Here's how the part is built. I have some questions about the finished solid (model axes, mm). A direction names the side the tool comes from. Coordinates: 2 decimals unless noted, no trailing zeros. Loops run counter-clockwise (first coordinate to the right, second up) from the corner with the lowest first, then second, coordinate; pieces in that order, holes last. Notation, with made-up numbers: (0.5, 73.5) -> (51.5, 73.5) arc R28 ccw to (51.5, 92.5) -> close; hole circle Ø8 at (88, 50.5). An arc over 180 degrees is marked (long way). Answer as a JSON object with one key per item and string values. Group by question number.
Q1. On a 3-axis mill with a long thin cutter (end or side, diameter ignored), from which of +Z, -Z, +X, -X, +Y, -Y can I reach the whole of each face in a straight line? I mean faces 5 (the cylindrical face through (-4.231, -4.254, 4.19)), 6 (the flat face through (-3, -3, 12.7)). Say none if no direction works.
Q2. I need wall thicknesses on line 1 (Y direction, x = 0, z = 22.9) (3 decimals); line 2 (Z direction, x = 1.75, y = -2.5); line 3 (Y direction, x = 2, z = 21.25). Which ranges of each line are inside material? Lowest first, please.
Q3. I'm going to push flat-ended pins straight in: pin 1 (4 mm diameter, centred on x = -2, z = 14.5, fed in from +Y); pin 2 (3 mm diameter, centred on y = -3, z = 15, fed in from +X); pin 3 (3 mm diameter, centred on x = -1, y = -1, fed in from -Z); pin 4 (2.5 mm diameter, centred on x = 0.5, y = 0.5, fed in from +Z). Where does each tip first touch, or does it pass through?
Q4. Thinking about a two-plate mould opening in X: for faces 1 (the flat face through (0, 0, 21)), 2 (the flat face through (0, 5, 4)), 3 (the conical face through (3.73, -3.71, 10.57)), 4 (the conical face through (-3.73, 3.71, 10.57)), which applies, released by +X, released by -X, zero draft, split by the parting line, or undercut?
Q5. I want a section at A-A on z = 3.5. Write out the boundary of the cut face in (x, y).
Autodesk Inventor part; units mm, degrees
ref_plane "Work Plane1" through (0, 0, 12.7) normal (0, 0, -1) x (-1, 0, 0)
ref_plane "YZ Plane" through (0, 0, 0) normal (1, 0, 0) x (0, 1, 0)
ref_plane "XZ Plane" through (0, 0, 0) normal (0, 1, 0) x (-1, 0, 0)
sketch "Sketch1" plane through (0, 0, 0) normal (0, 0, 1) x (1, 0, 0)
  circle A0 centre (0, 0) radius 6
  dimension "d0" = 12
extrude "Extrusion1" add sketch "Sketch1" along normal blind 24
sketch "Sketch2" plane through (0, 0, 0) normal (0, 0, -1) x (-1, 0, 0)
  line L0 (-5, -5) -> (5, -5)
  line L1 (5, -5) -> (5, 5)
  line L2 (5, 5) -> (-5, 5)
  line L3 (-5, 5) -> (-5, -5)
  line L4 (-5, -5) -> (5, 5) construction
  line L5 (5, -5) -> (-5, 5) construction
  circle A0 centre (0, 0) radius 7.723
  dimension "d3" = 10
  dimension "d4" = 10
extrude "Extrusion2" cut sketch "Sketch2" against normal blind 8.5
sketch "Sketch3" plane through (0, 0, 24) normal (0, 0, 1) x (1, 0, 0)
  circle A0 centre (0, 0) radius 3.175
  dimension "d7" = 6.35
extrude "Extrusion3" cut sketch "Sketch3" against normal blind 3
ref_plane "Work Plane1" through (0, 0, 12.7) normal (0, 0, -1) x (-1, 0, 0)
sketch "Sketch5" plane through (0, 0, 24) normal (0, 0, 1) x (1, 0, 0)
  circle A0 centre (0, 0) radius 3.96
  circle A1 centre (0, 0) radius 11.6408
  dimension "d14" = 7.92
extrude "Extrusion4" cut sketch "Sketch5" against normal up to surface (15.5 mm away)
sketch "Sketch6" plane through (-3.3166, 5, 8.5) normal (0, 0, 1) x (1, 0, 0)
  line L0 (8.3166, -1.6834) -> (8.3166, -8.3166)
  arc A0 (8.3166, -1.6834) -> (6.6332, 0) centre (3.3166, -5) ccw
  line L1 (0, 0) -> (6.6332, 0)
  arc A1 (0, 0) -> (-1.6834, -1.6834) centre (3.3166, -5) ccw
  line L2 (-1.6834, -8.3166) -> (-1.6834, -1.6834)
  arc A2 (-1.6834, -8.3166) -> (0, -10) centre (3.3166, -5) ccw
  line L3 (6.6332, -10) -> (0, -10)
  arc A3 (6.6332, -10) -> (8.3166, -8.3166) centre (3.3166, -5) ccw
  circle A4 centre (3.3166, -5) radius 3.96 construction
sketch "Sketch7" plane through (0, 0, 12.7) normal (0, 0, -1) x (-1, 0, 0)
  circle A0 centre (0, 0) radius 3.96 construction
  circle A1 centre (0, 0) radius 3.175 construction
  circle A2 centre (0, 0) radius 4.5
  dimension "d18" = 9
loft "Loft1" add profiles "Sketch6", "Sketch7"
properties part number "J0_Post"
Result set:
{
 "1": {"face 5": "+Z, -Z, -X, -Y", "face 6": "+Z"},
 "2": {"line 1": "y = -3.96 to -3.175, 3.175 to 3.96", "line 2": "z = 0 to 21", "line 3": "y = -3.42 to -2.47, 2.47 to 3.42"},
 "3": {"pin 1": "stops at y = 4.36", "pin 2": "stops at x = 3.66", "pin 3": "stops at z = 0", "pin 4": "stops at z = 21"},
 "4": {"face 1": "undercut", "face 2": "zero draft", "face 3": "released by +X", "face 4": "released by -X"},
 "5": {"outline": "(-5, -3.32) arc R6 ccw to (-3.32, -5) -> (3.32, -5) arc R6 ccw to (5, -3.32) -> (5, 3.32) arc R6 ccw to (3.32, 5) -> (-3.32, 5) arc R6 ccw to (-5, 3.32) -> close"}
}
